For this review, take the finished solid that the model builds, in its own axes (mm). Give positions to 0.01 mm unless a question says otherwise; leave off trailing zeros. Order: outer loops, then holes, each group sorted by start corner. A loop starts at its lowest first (then second) coordinate and runs counter-clockwise, first axis right, second up. Notation, with made-up numbers: (46.25, 51) - (52.25, 51) arc R21 ccw to (52.25, 79) - close; hole circle Ø6 at (-31, -12). An arc over 180 degrees is marked (long way). One line per item, written item: value.
```python
from build123d import *

# Parameters (mm, degrees)
SKETCH1_R               = 40.5
SKETCH1_R_2             = 2.5
BOSS_EXTRUDE1_DEPTH     = 4.7625
SWEEP_THIN1_PROFILE_R   = 12.3571
SWEEP_THIN1_PROFILE_R_2 = 11.1125
CUT_EXTRUDE2_DEPTH      = 96.807184511
CUT_EXTRUDE2_DEPTH_BACK = 96.807184511
SKETCH18_R              = 3


with BuildPart() as part:
    # Sketch1 → Boss-Extrude1 (new body)
    with BuildSketch(Plane.XY):
        with Locations(Location((0, 0, 0), (0, 0, 180))):
            Circle(SKETCH1_R)
        with Locations(Location((-30.310889132, -17.5, 0), (0, 0, 180))):
            Circle(SKETCH1_R_2, mode=Mode.SUBTRACT)
        with Locations(Location((0, -35, 0), (0, 0, 180))):
            Circle(SKETCH1_R_2, mode=Mode.SUBTRACT)
        with Locations(Location((30.310889132, -17.5, 0), (0, 0, 180))):
            Circle(SKETCH1_R_2, mode=Mode.SUBTRACT)
        with Locations(Location((30.310889132, 17.5, 0), (0, 0, 180))):
            Circle(SKETCH1_R_2, mode=Mode.SUBTRACT)
        with Locations(Location((0, 35, 0), (0, 0, 180))):
            Circle(SKETCH1_R_2, mode=Mode.SUBTRACT)
        with Locations(Location((-30.310889132, 17.5, 0), (0, 0, 180))):
            Circle(SKETCH1_R_2, mode=Mode.SUBTRACT)
    extrude(amount=BOSS_EXTRUDE1_DEPTH)

    # Sweep-Thin1: sweep along a path in Sketch6
    with BuildLine(Plane(origin=(0, 0, 0), x_dir=(0, 0, -1), z_dir=(1, 0, 0))) as sweep_thin1_path:
        Line((0, 0), (-73.603547963, -19.722011237))
    # Sweep-Thin1 profile (on start of the path) → Sweep-Thin1 (sweep)
    with BuildSketch(Plane(origin=(0, 0, 0), x_dir=(0, 0.965925826289069, 0.25881904510251813), z_dir=(0, -0.25881904510251813, 0.965925826289069))):
        Circle(SWEEP_THIN1_PROFILE_R)
        Circle(SWEEP_THIN1_PROFILE_R_2, mode=Mode.SUBTRACT)
    sweep(path=sweep_thin1_path.line)

    # Sketch18 → Cut-Extrude2 (cut, two sides: drawn at the far end of the back side and taken through both)
    with BuildSketch(Plane(origin=(0, 0, 0), x_dir=(-1, 0, 0), z_dir=(0, -0.9659258262890691, -0.25881904510251813)).offset(-CUT_EXTRUDE2_DEPTH_BACK)):
        with Locations(Location((0, -63.5, 0), (0, 0, 90))):
            Circle(SKETCH18_R)
        with Locations(Location((0, -50.8, 0), (0, 0, 90))):
            Circle(SKETCH18_R)
    extrude(amount=CUT_EXTRUDE2_DEPTH + CUT_EXTRUDE2_DEPTH_BACK, mode=Mode.SUBTRACT)


solid = part.part
```
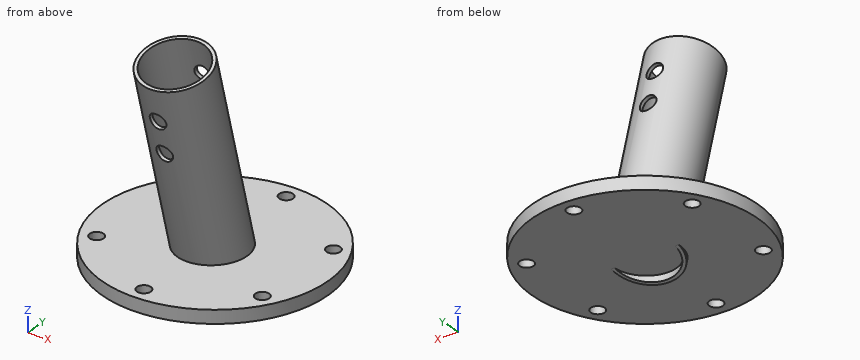
(1) Take a section at B-B (y = -35). Write out the cut boundary in (x, z), then the cut area to 3 significant figures.
Answers below:
outline: (-20.38, 0) - (-2.5, 0) - (-2.5, 4.76) - (-20.38, 4.76) - close; (2.5, 0) - (20.38, 0) - (20.38, 4.76) - (2.5, 4.76) - close
area: 170 mm^2
(2) Take a section at C-C (y = 17.5). Write out the cut boundary in (x, z), then the cut area to 3 significant figures.
Answers below:
outline: (-36.52, 0) - (-32.81, 0) - (-32.81, 4.76) - (-36.52, 4.76) - close; (-27.81, 0) - (27.81, 0) - (27.81, 4.76) - (-27.81, 4.76) - close; (32.81, 0) - (36.52, 0) - (36.52, 4.76) - (32.81, 4.76) - close
area: 300 mm^2
(3) For P1, Ø4, axis at x = 30.31, y = -17.5, coming from the +Z side; P2, Ø4, axis at y = -22, z = 39.5, coming from the +X side; P3, Ø2, axis at y = -5, z = 57, coming from the +X side; P4, Ø8, axis at x = -30.31, y = -17.5, coming from the -Z side, all flat-tipped, find the tip position at first contact; note any pin that passes through.
Answers below:
P1: passes through
P2: stops at x = 8.44
P3: stops at x = 8.55
P4: stops at z = 0
(4) Take a section at A-A (z = 3). Write out the cut boundary in (x, y).
Answers below:
outline: circle Ø81 at (0, 0); hole circle Ø5 at (-30.31, -17.5); hole circle Ø5 at (-30.31, 17.5); hole circle Ø5 at (0, -35); hole circle Ø5 at (0, 35); hole circle Ø5 at (30.31, -17.5); hole circle Ø5 at (30.31, 17.5)
(5) Take a section at D-D (y = -17.5). Give the number of separate pieces and of enclosed holes in the cut face, then the cut area to 3 significant figures.
Answers below:
separate pieces: 4
enclosed holes: 0
area: 500 mm^2
(6) Wall thickness on line 1 (Y direction, x = 0, z = 3); line 2 (X direction, y = 17, z = 3); line 3 (X direction, y = -14, z = 50): over which ranges is each line inside the solid? List them lowest first. Write a range as from..to.
Answers below:
line 1: y = -40.5..-37.5, -32.5..32.5, 37.5..40.5
line 2: x = -36.76..-32.76, -27.86..27.86, 32.76..36.76
line 3: x = -12.34..-11.1, 11.1..12.34
